Part model, mm, in its own coordinate system. Face numbers are marked on the shaded views. A direction names the side the tool comes from. Round coordinates to 2 decimals unless told otherwise and drop trailing zeros. Write each loop counter-clockwise with the first axis right and the second up, starting at its lowest first coordinate (ties: lowest second). Pieces come first, ordered by that corner, then holes. Notation, with made-up numbers: (83.5, 1) -> (92.5, 1) arc R27 ccw to (92.5, 18) -> close; hole circle Ø10 at (6, 25.25). An arc over 180 degrees is marked (long way). Return JSON: item names as keys, results as strings. Group by question number.
(1) Saw through at C-C (y = 0). List the corners of the cut face in (x, z), plus the area to 3 significant figures.
(2) Tool access for the marked faces 4, 5 and 6: list every direction of +Z, -Z, +X, -X, +Y, -Y with a clear straight run to the whole face (end or side of a thin tool).
(3) Mould opens along Y. For the marked faces 1, 2 and 3 say: +Y half, -Y half, draft (parallel to the pull), parting line (faces both ways), or undercut.
(4) Saw through at A-A (z = 48.5). List the corners of the cut face in (x, y), plus the area to 3 significant figures.
(5) Saw through at B-B (x = -22). List the corners of the cut face in (y, z), plus the area to 3 significant figures.
(6) Drill centre lines: L1, parallel to Z at x = -22, y = -33; L2, parallel to Y at x = -34, z = 63; L3, parallel to Z at x = -15, y = -4. Where is each one in solid material? Low to high. Write a range as from..to.
(7) Saw through at D-D (z = 25.5). List the corners of the cut face in (x, y).
(8) Drop flat-ended pins along their axis: pin 1 Ø17.5 at (y, z) = (-29.5, 51.5) entering from -X; pin 2 Ø12 at (x, z) = (-22, 68) entering from +Y; pin 3 Ø9.5 at (x, y) = (-89.5, -8) entering from +Z; pin 4 Ø4 at (x, y) = (-32, -22.5) entering from +Z. Give the stop position or say it passes through.
from build123d import *

# Parameters (mm, degrees)
F0_R     = 10
F1_DEPTH = 40
F2_DEPTH = 24
F4_DEPTH = 10


with BuildPart() as f1:
    # F0 (on Front) → F1 (new body, symmetric)
    with BuildSketch(Plane.XZ):
        Polygon((-100, 0), (0, 0), (0, 30), (-44, 30), (-100, 30), align=None)
        with BuildLine():
            Line((-44, 30), (0, 30))
            Line((0, 30), (0, 68))
            ThreePointArc((0, 68), (-22, 90), (-44, 68))
            Line((-44, 68), (-44, 30))
        make_face()
        with Locations((-22, 68)):
            Circle(F0_R, mode=Mode.SUBTRACT)
    extrude(amount=F1_DEPTH, both=True)

    # F0 (on Front) → F2 (cut, symmetric)
    with BuildSketch(Plane.XZ):
        with BuildLine():
            Line((-44, 30), (0, 30))
            Line((0, 30), (0, 68))
            ThreePointArc((0, 68), (-22, 90), (-44, 68))
            Line((-44, 68), (-44, 30))
        make_face()
        with Locations((-22, 68)):
            Circle(F0_R, mode=Mode.SUBTRACT)
    extrude(amount=F2_DEPTH, both=True, mode=Mode.SUBTRACT)

    # F3 (on face) → F4 (cut)
    with BuildSketch(Plane.XY.offset(30)):
        with BuildLine():
            Line((-100, -16), (-76, -16))
            ThreePointArc((-76, -16), (-60, 0), (-76, 16))
            Line((-76, 16), (-100, 16))
            Line((-100, 16), (-100, 8.16))
            Line((-100, 8.16), (-76, 8.16))
            ThreePointArc((-76, 8.16), (-67.84, 0), (-76, -8.16))
            Line((-76, -8.16), (-100, -8.16))
            Line((-100, -8.16), (-100, -16))
        make_face()
    extrude(amount=-F4_DEPTH, mode=Mode.SUBTRACT)


solid = f1.part
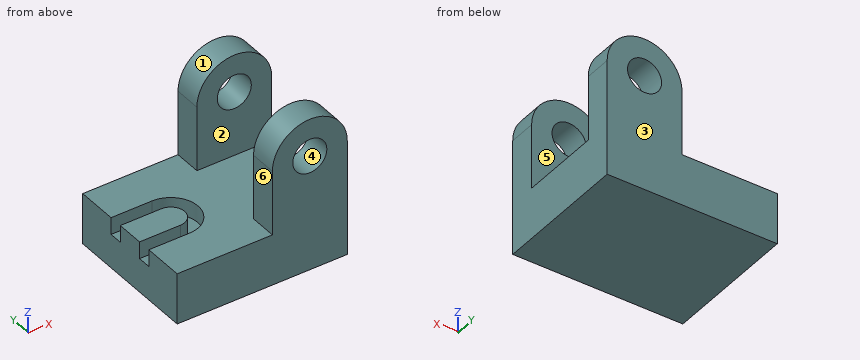
Computed values:
{
 "1": {"outline": "(-100, 0) -> (0, 0) -> (0, 30) -> (-60, 30) -> (-60, 20) -> (-67.84, 20) -> (-67.84, 30) -> (-100, 30) -> close", "area": "2,920 mm2"},
 "2": {"face 4": "+Y, -Y", "face 5": "+Z, +X, -X", "face 6": "+Z, -X, +Y, -Y"},
 "3": {"face 1": "draft", "face 2": "undercut", "face 3": "+Y half"},
 "4": {"outline": "(-44, -40) -> (0, -40) -> (0, -24) -> (-44, -24) -> close; (-44, 24) -> (0, 24) -> (0, 40) -> (-44, 40) -> close", "area": "1,410 mm2"},
 "5": {"outline": "(-40, 0) -> (40, 0) -> (40, 58) -> (24, 58) -> (24, 30) -> (-24, 30) -> (-24, 58) -> (-40, 58) -> close; (-40, 78) -> (-24, 78) -> (-24, 90) -> (-40, 90) -> close; (24, 78) -> (40, 78) -> (40, 90) -> (24, 90) -> close", "area": "3,680 mm2"},
 "6": {"L1": "0..58, 78..90", "L2": "-40..-24, 24..40", "L3": "0..30"},
 "7": {"outline": "(-100, -40) -> (0, -40) -> (0, 40) -> (-100, 40) -> (-100, 16) -> (-76, 16) arc R16 cw to (-76, -16) -> (-100, -16) -> close; (-100, -8.16) -> (-76, -8.16) arc R8.16 ccw to (-76, 8.16) -> (-100, 8.16) -> close"},
 "8": {"pin 1": "x = -44", "pin 2": "through", "pin 3": "z = 30", "pin 4": "z = 88.22"}
}
